from build123d import *

# Parameters (mm, degrees)
F0_W     = 55.290274322
F0_H     = 83.3742246032
F1_DEPTH = 25.4
F2_R     = 15.8926372782
F3_DEPTH = 25.401
F4_W     = 11.2183341355
F4_H     = 57.9742246032
F5_DEPTH = 19.05
F7_DEPTH = 19.05
F8_R     = 5.08


# Not quite as in the source:
# - a pattern or mirror of a feature is missing from the dataset's text; its kind, count and spacing are read off the source's solid


with BuildPart() as f1:
    # F0 (on Top) → F1 (new body)
    with BuildSketch(Plane.XY):
        Rectangle(F0_W, F0_H)
    extrude(amount=F1_DEPTH)

    # F2 (on face) → F3 (cut, through all)
    with BuildSketch(Plane.XY.offset(25.4)):
        with Locations((27.645137161, 0)):
            Circle(F2_R)
    extrude(amount=-F3_DEPTH, mode=Mode.SUBTRACT)

    # F4 (on face) → F5 (cut)
    with BuildSketch(Plane.XY.offset(25.4)):
        with Locations((-22.0359700932, 0)):
            Rectangle(F4_W, F4_H)
    extrude(amount=-F5_DEPTH, mode=Mode.SUBTRACT)

    # F6 (on face) → F7 (cut)
    with BuildSketch(Plane.XY.offset(25.4)):
        with BuildLine():
            Line((27.645137161, -41.6871123016), (27.645137161, -19.3835441023))
            Line((27.645137161, -19.3835441023), (10.0954379886, -19.3835441023))
            ThreePointArc((10.0954379886, -19.3835441023), (3.1118668584, -20.9577512479), (0, -27.4048186839))
            Line((0, -27.4048186839), (0, -35.3843905032))
            Line((0, -35.3843905032), (-27.645137161, -35.3843905032))
            Line((-27.645137161, -35.3843905032), (-27.645137161, -41.6871123016))
            Line((-27.645137161, -41.6871123016), (27.645137161, -41.6871123016))
        make_face()
    f7 = extrude(amount=-F7_DEPTH, mode=Mode.SUBTRACT)

    # F7_copies: F7 across plane
    add(f7.mirror(Plane.ZX), mode=Mode.SUBTRACT)

    # F8
    f8_edges = [f1.edges().sort_by_distance(p)[0] for p in [
        (27.645137, -41.687112, 3.175),
        (27.645137, 41.687112, 3.175),
        (-27.645137, 41.687112, 3.175),
        (-27.645137, -41.687112, 3.175),
    ]]
    fillet(f8_edges, radius=F8_R)


solid = f1.part
For this review, take the finished solid that the model builds, in its own axes (mm). A direction names the side the tool comes from. Give positions to 0.01 mm unless a question says otherwise; leave off trailing zeros. Order: outer loops, then holes, each group sorted by start corner. A loop starts at its lowest first (then second) coordinate and runs counter-clockwise, first axis right, second up. Notation, with made-up numbers: (-4.75, 5.5) -> (11.25, 5.5) arc R15 ccw to (11.25, 32.5) -> close; hole circle Ø10 at (70.25, 83.5). An arc over 180 degrees is marked (long way). Write item = value, one per line.
1) We need section C-C, the plane x = -14. Give the boundary of the cut face in (y, z).
Findings:
outline = (-41.69, 0) -> (41.69, 0) -> (41.69, 6.35) -> (35.38, 6.35) -> (35.38, 25.4) -> (-35.38, 25.4) -> (-35.38, 6.35) -> (-41.69, 6.35) -> close
2) We need section D-D, the plane y = 0. Give the boundary of the cut face in (x, z).
Findings:
outline = (-27.65, 0) -> (11.75, 0) -> (11.75, 25.4) -> (-16.43, 25.4) -> (-16.43, 6.35) -> (-27.65, 6.35) -> close
3) For faces 1 (the face through (19, 19.384, 16)), 2 (the face through (3.193, -20.894, 16.008)), 3 (the face through (-16.427, 0, 16)), 4 (the face through (19, -19.384, 16)), 5 (the face through (27.645, -25, 6)), list the 3-axis set-ups (+Z, -Z, +X, -X, +Y, -Y) from which the entire face can be reached by the end or side of a thin tool; tool diameter is ignored.
Findings:
face_1 = +Z, +X, +Y
face_2 = +Z, -Y
face_3 = +Z, -X
face_4 = +Z, +X, -Y
face_5 = +Z, -Z, +X, +Y, -Y
4) We need section B-B, the plane x = 20. Give the boundary of the cut face in (y, z), and give its area (3 significant figures).
Findings:
outline = (-41.69, 0) -> (-13.93, 0) -> (-13.93, 25.4) -> (-19.38, 25.4) -> (-19.38, 6.35) -> (-41.69, 6.35) -> close; (13.93, 0) -> (41.69, 0) -> (41.69, 6.35) -> (19.38, 6.35) -> (19.38, 25.4) -> (13.93, 25.4) -> close
area = 560 mm^2
5) Insertion check: pin 1 (4 mm diameter, centred on x = -21.5, z = 6.5, fed in from +Y); pin 2 (12.5 mm diameter, centred on x = -21.5, z = 16, fed in from +Y); pin 3 (9.5 mm diameter, centred on y = 12.5, z = 20.5, fed in from -X); pin 4 (5 mm diameter, centred on y = -5.5, z = 17.5, fed in from +X). Each pin has a flat end and moves straight along its axis. Give the tip position at first contact, or say it passes through.
Findings:
pin_1 = 41.69
pin_2 = 35.38
pin_3 = -16.43
pin_4 = 13.91
6) We need section A-A, the plane z = 22.5. Give the boundary of the cut face in (x, y), and give its area (3 significant figures).
Findings:
outline = (-27.65, -35.38) -> (0, -35.38) -> (0, -27.4) arc R8.23 cw to (10.1, -19.38) -> (27.65, -19.38) -> (27.65, -15.89) arc R15.89 cw to (27.65, 15.89) -> (27.65, 19.38) -> (10.1, 19.38) arc R8.23 cw to (0, 27.4) -> (0, 35.38) -> (-27.65, 35.38) -> (-27.65, 28.99) -> (-16.43, 28.99) -> (-16.43, -28.99) -> (-27.65, -28.99) -> close
area = 2,010 mm^2
7) To check wall thickness, follow L1, parallel to Y at x = -24, z = 21.5; L2, parallel to Y at x = -12.5, z = 16.25; L3, parallel to X at y = -35, z = 11. State the ranges of each line that lie inside material, in increasing order. Write a range as from..to.
Findings:
L1 = -35.38..-28.99, 28.99..35.38
L2 = -35.38..35.38
L3 = -27.65..0
8) Draft analysis for pull direction Y (two halves, no side actions). For faces 6 (the face through (-22, -28.987, 16)), 7 (the face through (-14, 35.384, 16)), 8 (the face through (-14, -35.384, 16)), 9 (the face through (-22, 0, 6.35)), state which applies: pulls with the +Y half, pulls with the -Y half, needs draft (parallel to the pull), parting line crosses it, or undercut.
Findings:
face_6 = undercut
face_7 = pulls with the +Y half
face_8 = pulls with the -Y half
face_9 = undercut
